from build123d import *

# Parameters (mm, degrees)
BOSS_EXTRUDE1_DEPTH = 10
SKETCH2_R           = 7.5
BOSS_EXTRUDE2_DEPTH = 56
SKETCH3_W           = 20
SKETCH3_H           = 20
BOSS_EXTRUDE3_DEPTH = 8


with BuildPart() as part:
    # Sketch1 → Boss-Extrude1 (new body)
    with BuildSketch(Plane.XY):
        with BuildLine():
            Line((-28.618176043, 41), (-14.309088021, -4.5))
            ThreePointArc((-14.309088021, -4.5), (0, -15), (14.309088021, -4.5))
            Line((14.309088021, -4.5), (28.618176042, 41))
            ThreePointArc((28.618176042, 41), (0, 80), (-28.618176043, 41))
        make_face()
    extrude(amount=BOSS_EXTRUDE1_DEPTH)

    # Sketch2 → Boss-Extrude2 (add)
    with BuildSketch(Plane.XY.offset(10)):
        with Locations((0, 50)):
            Circle(SKETCH2_R)
    extrude(amount=BOSS_EXTRUDE2_DEPTH)

    # Sketch3 → Boss-Extrude3 (add)
    with BuildSketch(Plane.XY.offset(66)):
        with Locations((0, 50)):
            Rectangle(SKETCH3_W, SKETCH3_H)
    extrude(amount=BOSS_EXTRUDE3_DEPTH)


solid = part.part
Geometry check sheet. Reference: the model listing, model coordinates, mm. A direction names the side the tool comes from. Round coordinates to 2 decimals unless told otherwise and drop trailing zeros. Write each loop counter-clockwise with the first axis right and the second up, starting at its lowest first coordinate (ties: lowest second). Pieces come first, ordered by that corner, then holes.
Item 1: Go/stop test with flat-tipped pins: pin 1 Ø6.5 at (y, z) = (54, 71) entering from -X; pin 2 Ø9 at (x, z) = (-3, 68) entering from -Y; pin 3 Ø10 at (x, y) = (3.5, 46.5) entering from -Z; pin 4 Ø3 at (x, y) = (-4, 31.5) entering from +Z. Record where each tip stops, or that it passes through.
Determined:
pin 1: stops at x = -10
pin 2: stops at y = 40
pin 3: stops at z = 0
pin 4: stops at z = 10
Item 2: Mould release check, pull along Z, two halves, no side actions. Record for faces 1 (the face through (21.363, 17.932, 4.93)), 2 (the face through (0, 33, 0)), 3 (the face through (4, 57, 66)), 4 (the face through (-1.63, 42.68, 37.61)): +Z half, -Z half, draft (parallel to the pull), parting line (faces both ways), or undercut.
Determined:
face 1: draft
face 2: -Z half
face 3: undercut
face 4: undercut
Item 3: Section check D-D (x = -24). Record the boundary of the cut face in (y, z), plus the area to 3 significant figures.
Determined:
outline: (26.32, 0) - (68, 0) - (68, 10) - (26.32, 10) - close
area: 417 mm2
Item 4: Section check C-C (z = 34.5). Record the boundary of the cut face in (x, y), plus the area to 3 significant figures.
Determined:
outline: circle Ø15 at (0, 50)
area: 177 mm2
Item 5: Access from +Z, -Z, +X, -X, +Y, -Y to the whole of each face (thin tool, end or side, straight path). Record for faces 5 (the face through (0, 40, 70)), 6 (the face through (10, 50, 70)), 7 (the face through (-21.564, 18.568, 4.93)), 8 (the face through (0, 60, 70)), 9 (the face through (-10, 50, 70)).
Determined:
face 5: +Z, +X, -X, -Y
face 6: +Z, +X, +Y, -Y
face 7: +Z, -Z, -X, -Y
face 8: +Z, +X, -X, +Y
face 9: +Z, -X, +Y, -Y
Item 6: Section check B-B (y = 50). Record the boundary of the cut face in (x, z).
Determined:
outline: (-30, 0) - (30, 0) - (30, 10) - (7.5, 10) - (7.5, 66) - (10, 66) - (10, 74) - (-10, 74) - (-10, 66) - (-7.5, 66) - (-7.5, 10) - (-30, 10) - close
Item 7: Material ranges on line 1 along Z through (x, y) = (0, -6); line 2 along Y through (x, z) = (-0.5, 66.5); line 3 along X through (y, z) = (44, 12.5), recorded low to high.
Determined:
line 1: z = 0 to 10
line 2: y = 40 to 60
line 3: x = -4.5 to 4.5
Item 8: Section check A-A (x = 0). Record the boundary of the cut face in (y, z).
Determined:
outline: (-15, 0) - (80, 0) - (80, 10) - (57.5, 10) - (57.5, 66) - (60, 66) - (60, 74) - (40, 74) - (40, 66) - (42.5, 66) - (42.5, 10) - (-15, 10) - close
